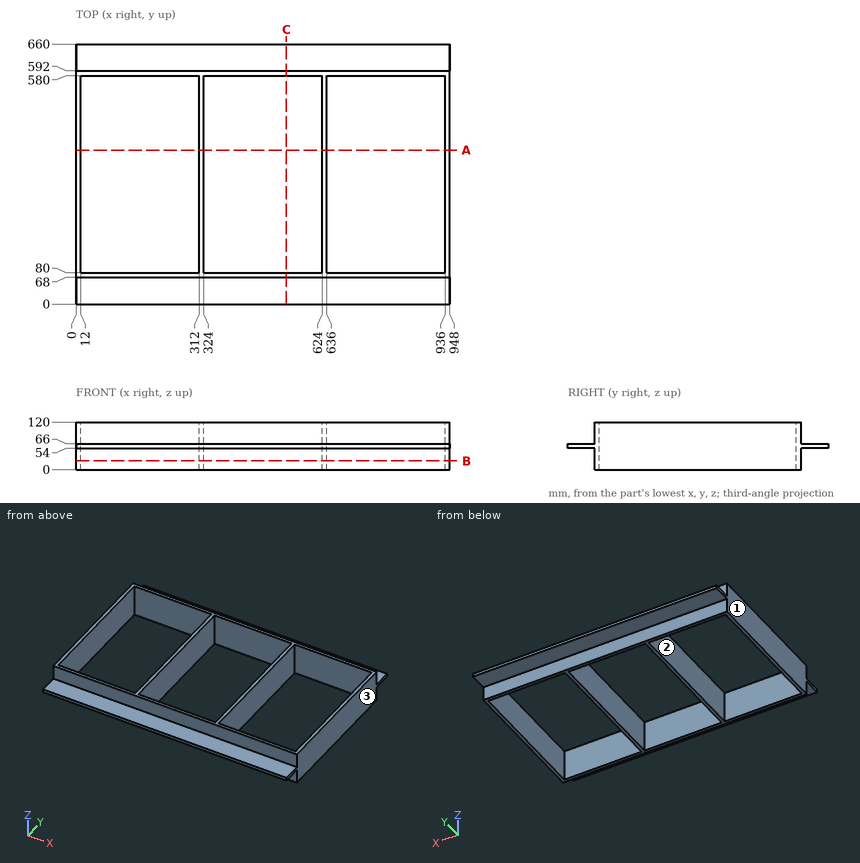
The drawing under review shows one solid part. Ordinate dimensions are in mm from its lowest x, y, z. Round coordinates to 2 decimals unless told otherwise and drop trailing zeros. Order: outer loops, then holes, each group sorted by start corner. A loop starts at its lowest first (then second) coordinate and runs counter-clockwise, first axis right, second up. Notation, with made-up numbers: (-5, 32.25) -> (4, 32.25) arc R20 cw to (4, 51.25) -> close; hole circle Ø3 at (44.25, -27). An arc over 180 degrees is marked (long way). Use a Markdown table: item, result.
Q1. For line 1 (X direction, y = 320, z = 48); line 2 (Y direction, x = 242, z = 25); line 3 (Z direction, x = 356, y = 593), list the stretches that pass through material, from the lowest coordinate up.
Values:
| item | result |
|---|---|
| line 1 | x = 0 to 12, 312 to 324, 624 to 636, 936 to 948 |
| line 2 | y = 68 to 80, 580 to 592 |
| line 3 | z = 54 to 66 |
Q2. Mouldability with a two-part tool opening along X and no side actions: class the marked faces 1, 2 and 3 as +X half, -X half, draft (parallel to the pull), parting line (faces both ways), or undercut.
Values:
| item | result |
|---|---|
| face 1 | -X half |
| face 2 | undercut |
| face 3 | +X half |
Q3. We need section C-C on x = 533.5. Write out the cut boundary in (y, z).
Values:
| item | result |
|---|---|
| outline | (0, 54) -> (68, 54) -> (68, 0) -> (80, 0) -> (80, 120) -> (68, 120) -> (68, 66) -> (0, 66) -> close; (580, 0) -> (592, 0) -> (592, 54) -> (660, 54) -> (660, 66) -> (592, 66) -> (592, 120) -> (580, 120) -> close |
Q4. We need section A-A on y = 391. Write out the cut boundary in (x, z), then the cut area to 3 significant figures.
Values:
| item | result |
|---|---|
| outline | (0, 0) -> (12, 0) -> (12, 120) -> (0, 120) -> close; (312, 0) -> (324, 0) -> (324, 120) -> (312, 120) -> close; (624, 0) -> (636, 0) -> (636, 120) -> (624, 120) -> close; (936, 0) -> (948, 0) -> (948, 120) -> (936, 120) -> close |
| area | 5,760 mm^2 |
Q5. Clearance check with flat-ended pins moving along their axes: P1, Ø12, axis at x = 558, z = 20.5, coming from the +Y side; P2, Ø1, axis at x = 567, z = 102, coming from the -Y side. State where each tip first meets the part, or that it passes through.
Values:
| item | result |
|---|---|
| P1 | stops at y = 592 |
| P2 | stops at y = 68 |
Q6. We need section B-B on z = 22. Write out the cut boundary in (x, y), then the cut area to 3 significant figures.
Values:
| item | result |
|---|---|
| outline | (0, 68) -> (948, 68) -> (948, 592) -> (0, 592) -> close; hole (12, 80) -> (312, 80) -> (312, 580) -> (12, 580) -> close; hole (324, 80) -> (624, 80) -> (624, 580) -> (324, 580) -> close; hole (636, 80) -> (936, 80) -> (936, 580) -> (636, 580) -> close |
| area | 46,800 mm^2 |
